from build123d import *

# Parameters (mm, degrees)
BOSS_EXTRUDE1_DEPTH = 7
CIRPATTERN1_COUNT   = 20
SKETCH4_R           = 7.5
SKETCH4_R_2         = 6.75
CUT_EXTRUDE1_DEPTH  = 7


with BuildPart() as part:
    # Sketch2 → Revolve1 (revolve)
    with BuildSketch(Plane.XY, mode=Mode.PRIVATE) as revolve1_sk:
        Polygon((-2.5, 0), (-8, 0), (-8, 7.1), (-6.11, 7.1), (-6.11, 14.1), (-8, 14.1), (-8, 16), (-2.5, 16), align=None)
    revolve(revolve1_sk.sketch.rotate(Axis((0, 0, 0), (0, 1, 0)), 270), axis=Axis((0, 0, 0), (0, 1, 0)))

    # Sketch3 → Boss-Extrude1 (add)
    with BuildSketch(Plane(origin=(0, 7.1, 0), x_dir=(1, 0, 0), z_dir=(0, 1, 0))):
        Polygon((-6, 1), (-6, -1), (-7, 0), align=None)
    boss_extrude1 = extrude(amount=BOSS_EXTRUDE1_DEPTH)

    # CirPattern1: Boss-Extrude1 ×20 about axis
    cirpattern1_axis = Axis((0, 0, 0), (0, 1, 0))
    for i in range(1, CIRPATTERN1_COUNT):
        add(boss_extrude1.rotate(cirpattern1_axis, i * 360 / CIRPATTERN1_COUNT))

    # Sketch4 → Cut-Extrude1 (cut)
    with BuildSketch(Plane(origin=(0, 7.1, 0), x_dir=(1, 0, 0), z_dir=(0, 1, 0))):
        Circle(SKETCH4_R)
        Circle(SKETCH4_R_2, mode=Mode.SUBTRACT)
    extrude(amount=CUT_EXTRUDE1_DEPTH, mode=Mode.SUBTRACT)


solid = part.part
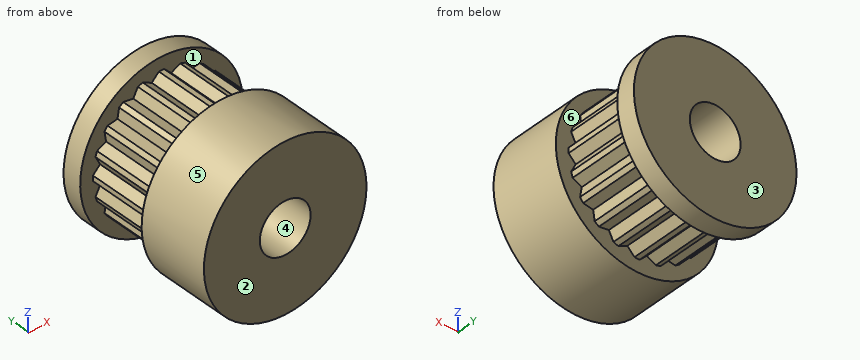
Could you check a few things on this model? Use its own coordinates, in mm. Face numbers are marked on the shaded views. A direction names the side the tool comes from. Give positions to 0.01 mm unless a question says otherwise; leave off trailing zeros. Order: outer loops, then holes, each group sorted by start corner. A loop starts at its lowest first (then second) coordinate and runs counter-clockwise, first axis right, second up. Notation, with made-up numbers: (-4, 55.25) -> (12, 55.25) arc R22 cw to (12, 61.25) -> close; hole circle Ø11 at (15.25, 53.5). An arc over 180 degrees is marked (long way). Return JSON: item names as keys, results as strings.
1. Imagine slicing it at A-A on z = 0. List the corners of the cut face in (x, y) for me, then the cut area to 4 significant figures.
Answer list:
{"outline": "(-8, 0) -> (-2.5, 0) -> (-2.5, 16) -> (-8, 16) -> (-8, 14.1) -> (-6.75, 14.1) -> (-6.75, 7.1) -> (-8, 7.1) -> close; (2.5, 0) -> (8, 0) -> (8, 7.1) -> (6.75, 7.1) -> (6.75, 14.1) -> (8, 14.1) -> (8, 16) -> (2.5, 16) -> close", "area": "158.5 mm2"}
2. I need wall thicknesses on line 1 (Y direction, x = 2.5, z = -7); line 2 (X direction, y = 6.75, z = 0); line 3 (X direction, y = 9.75, z = 0). Which ranges of each line are inside material? Lowest first, please. Write a range as from..to.
Answer list:
{"line 1": "y = 0..7.1, 14.1..16", "line 2": "x = -8..-2.5, 2.5..8", "line 3": "x = -6.75..-2.5, 2.5..6.75"}
3. Thinking about a two-plate mould opening in Y: for the marked faces 1, 2, 3 and 4, which applies, pulls with the +Y half, pulls with the -Y half, needs draft (parallel to the pull), parting line crosses it, or undercut?
Answer list:
{"face 1": "undercut", "face 2": "pulls with the -Y half", "face 3": "pulls with the +Y half", "face 4": "needs draft"}
4. On a 3-axis mill with a long thin cutter (end or side, diameter ignored), from which of +Z, -Z, +X, -X, +Y, -Y can I reach the whole of each face in a straight line? I mean the marked faces 5 and 6. Say none if no direction works.
Answer list:
{"face 5": "+Y, -Y", "face 6": "none"}
5. Imagine slicing it at C-C on y = 15.25. List the corners of the cut face in (x, z) for me, then the cut area to 3 significant figures.
Answer list:
{"outline": "circle Ø16 at (0, 0); hole circle Ø5 at (0, 0)", "area": "181 mm2"}
6. Imagine slicing it at B-B on x = 0. List the corners of the cut face in (y, z) for me.
Answer list:
{"outline": "(0, -8) -> (7.1, -8) -> (7.1, -6.75) -> (14.1, -6.75) -> (14.1, -8) -> (16, -8) -> (16, -2.5) -> (0, -2.5) -> close; (0, 2.5) -> (16, 2.5) -> (16, 8) -> (14.1, 8) -> (14.1, 6.75) -> (7.1, 6.75) -> (7.1, 8) -> (0, 8) -> close"}
7. For pin 1 Ø2 at (x, y) = (2.5, 9) entering from +Z; pin 2 Ø5 at (x, y) = (3, 5) entering from -Z; pin 3 Ø4 at (y, z) = (8, -3) entering from -X, each with a flat end and sliding along its axis, tell me the tip position at first contact or that it passes through.
Answer list:
{"pin 1": "stops at z = 6.49", "pin 2": "stops at z = -7.98", "pin 3": "stops at x = -7.91"}
